Autodesk Inventor part; units mm, degrees
ref_plane "Work Plane1" through (3, 0, 0) normal (0, 0.5, 0.8660254) x (1, 0, 0)
ref_plane "YZ Plane" through (0, 0, 0) normal (1, 0, 0) x (0, 1, 0)
ref_plane "XZ Plane" through (0, 0, 0) normal (0, 1, 0) x (-1, 0, 0)
sketch "Sketch1" plane through (0, 0, 0) normal (0, 0, 1) x (1, 0, 0)
  line L0 (0, 4) -> (0, 0)
  line L1 (0, 0) -> (40, 0)
  line L2 (40, 0) -> (40, 4)
  line L3 (40, 4) -> (0, 4)
  line L4 (-8, 0) -> (48, 0)
  line L5 (0, -0.8) -> (0, 4.8)
  dimension "d0" = 8
  dimension "d1" = 40
revolve "Body" add sketch "Sketch1" angle 360 about axis through (0, 0, 0) along (1, 0, 0)
sketch "Sketch2" plane through (0, 0, 0) normal (1, 0, 0) x (0, 1, 0)
  line L0 (0, 7.5056) -> (6.5, 3.7528)
  line L1 (6.5, 3.7528) -> (6.5, -3.7528)
  line L2 (6.5, -3.7528) -> (0, -7.5056)
  line L3 (0, -7.5056) -> (-6.5, -3.7528)
  line L4 (-6.5, -3.7528) -> (-6.5, 3.7528)
  line L5 (-6.5, 3.7528) -> (0, 7.5056)
  line L6 (-9.1, 0) -> (9.1, 0)
  line L7 (0, -10.5078) -> (0, 10.5078)
  point P0 (0, 0)
  point P1 (0, 0)
  dimension "d2" = 13
extrude "Head" add sketch "Sketch2" against normal blind 6.5
sketch "Sketch3" plane through (-6.5, 0, 0) normal (-1, 0, 0) x (0, 1, 0)
  circle A0 centre (0, 0) radius 4.875
  point P0 (0, 0)
  dimension "d12" = 9.75
extrude "Indent1" cut sketch "Sketch3" against normal blind 1.3
sketch "Sketch4" plane through (0, 0, 0) normal (0, 0, 1) x (1, 0, 0)
  line L0 (-6.5, 7.5056) -> (-6.5, 6.5)
  line L1 (-6.5, 6.5) -> (-5.9194, 7.5056)
  line L2 (-5.9194, 7.5056) -> (-6.5, 7.5056)
  line L3 (0, 7.5056) -> (0, 6.5)
  line L4 (0, 6.5) -> (-0.5806, 7.5056)
  line L5 (-0.5806, 7.5056) -> (0, 7.5056)
  line L6 (0, 0) -> (-6.5, 0)
  line L7 (-6.5, 0) -> (-6.5, 6.5)
  line L8 (0, 0) -> (0, 6.5)
  line L9 (-7.8, 0) -> (1.3, 0)
  line L10 (-5.9194, 7.5056) -> (-0.5806, 7.5056) construction
  line L11 (0, -1.5011) -> (0, 9.0067)
  dimension "d6" = 30
  dimension "d7" = 30
  dimension "d16" = 13
  dimension "d17" = 13
  dimension "d18" = 15.0111
revolve "Chamfer1" cut sketch "Sketch4" angle 360 about axis through (-10, 0, 0) along (1, 0, 0)
fillet "Fillet1" radius 0.4 1 edges at (0, -4, 0)
thread "Thread"
ref_plane "Work Plane1" through (3, 0, 0) normal (0, 0.5, 0.8660254) x (1, 0, 0)
equation "\"d2\" = SW"
equation "\"d3\" = KOH"
equation "\"d12\" = 0.75 * SW0"
equation "\"d14\" = 0.2 * KOH"
equation "\"d11\" = RR"
equation "\"d8\" = GEL"
equation "\"d0\" = GD"
equation "\"d1\" = NLG"
equation "\"d6\" = ANG1"
equation "\"d7\" = ANG1"
equation "\"d16\" = SW0"
equation "\"d17\" = SW0"
equation "\"d18\" = 1.1547 * SW"
equation "\"NLG\" = 40"
equation "\"KOH\" = 6.5"
equation "\"GD\" = NND"
equation "\"GEL\" = 37.5"
equation "\"SW\" = 13"
equation "\"SW0\" = SW"
equation "\"ANG1\" = 30deg"
equation "\"RR\" = 0.4"
equation "\"GUL\" = 0.61345 * PTC"
equation "\"SPD\" = NND - 1.2269 * PTC"
equation "\"GD1\" = THREADDIA - 1.2269 * PTC"
equation "\"THREADDIA\" = 8"
equation "\"SDH\" = 9.2"
equation "\"TOA\" = 30deg"
equation "\"BDM\" = NND"
equation "\"FAWI\" = 45deg"
equation "\"PTC\" = 1.25"
equation "\"NND\" = 8"
equation "\"GAL\" = 0.61345 * PTC"
equation "\"SD\" = 0"
equation "\"SD2\" = SDH"
equation "\"E0\" = 1.155 * SW"
properties part number "AS 1427 - M8 x 40" material "Steel, Mild"
The listing builds one solid part. Answer for the finished solid, in the listing's coordinates (mm). A direction names the side the tool comes from. Coordinates: 2 decimals unless noted, no trailing zeros. Write each loop counter-clockwise with the first axis right and the second up, starting at its lowest first coordinate (ties: lowest second). Pieces come first, ordered by that corner, then holes. Notation, with made-up numbers: M 62.25,-15.5 L 92.25,-15.5 A6 ccw 92.25,-6.5 Z; hole C -9.75,67.25 d11. An arc over 180 degrees is marked long. Use one line per item in the form item = value.
Item 1: Find section A-A, the plane x = 16. Give the vertices of the cut face in (y, z).
Model answer:
outline = C 0,0 d8
Item 2: Find the intervals of material crossed by probe 1 along Y at (x, z) = (-6.2, 0) (3 decimals); probe 2 along Z at (x, y) = (-5.65, 0) (3 decimals); probe 3 along X at (y, z) = (-4, -2.5), in increasing order.
Model answer:
probe_1 = -6.5 to -4.875, 4.875 to 6.5
probe_2 = -7.506 to -4.875, 4.875 to 7.506
probe_3 = -5.2 to 0
Item 3: For faces 1 (the face through (-0.12, -0.02, 6.71)), 2 (the face through (19.923, -0.867, 3.905)), determine the directions among +Z, -Z, +X, -X, +Y, -Y from which every point of the face is accessible in a straight line to the end or side of a thin tool.
Model answer:
face_1 = +Z, +X
face_2 = +X
Item 4: Given P1, Ø1, axis at x = 12.5, z = 0, coming from the -Y side; P2, Ø8, axis at x = 8, z = -5, coming from the +Y side; P3, Ø5, axis at y = 1, z = 1, coming from the -X side; P4, Ø1, axis at y = 4, z = 1.5, coming from the +X side, each flat-ended and moving along its own axis, determine where each tip first touches the part or whether it passes through.
Model answer:
P1 = -4
P2 = 3.87
P3 = -5.2
P4 = 40
Item 5: The mould has two halves that part along Z. Classify faces 3 (the face through (-6.5, 1, 5)), 4 (the face through (-3.2, 3.2, 5.66)), 5 (the face through (-0.12, -5.8, -3.37)), 6 (the face through (-5.859, -0.635, -4.834)): released by +Z, released by -Z, zero draft, split by the parting line, or undercut.
Model answer:
face_3 = zero draft
face_4 = released by +Z
face_5 = released by -Z
face_6 = undercut
